Model file for the job. Use its own axes, mm. A direction names the side the tool comes from. Give positions to 0.01 mm unless a question says otherwise; leave off trailing zeros. Loops run counter-clockwise (first coordinate to the right, second up) from the corner with the lowest first, then second, coordinate; pieces in that order, holes last. Notation, with made-up numbers: (-34.5, 72.5) - (16.5, 72.5) arc R31 ccw to (16.5, 109.5) - close; hole circle Ø1 at (9, -8). An arc over 180 degrees is marked (long way). Answer as CSV lines item,"result". Start each with the question number.
Item 1: Pull direction X, two halves, no side cores. Call faces 4 (the flat face through (0.25, 8, 1.6)), 5 (the cylindrical face through (-2.723, -0.637, 5.507)), 6 (the cylindrical face through (8, -1.72, 4.15)), 7 (the flat face through (1, 1, 6)): pulls with the +X half, pulls with the -X half, needs draft (parallel to the pull), parting line crosses it, or undercut.
Item 2: Drill centre lines: L1, parallel to Z at x = -0.75, y = -3; L2, parallel to X at y = -1.75, z = 3.1; L3, parallel to Y at x = 2, z = 4.4. Where is each one in solid material? Low to high. Write a range as from..to.
Item 3: Pin check, flat tips, straight feed: pin 1 (3 mm diameter, centred on y = 6, z = 2.5, fed in from +X); pin 2 (1 mm diameter, centred on x = 1, z = 2.5, fed in from -Y); pin 3 (5 mm diameter, centred on x = -1, y = -2, fed in from +Z); pin 4 (1 mm diameter, centred on y = 2, z = 3, fed in from +X). Stop position of each tip, or through.
Item 4: Saw through at A-A on y = 6.75. Give the cut face in (x, z), plus the area to 3 significant figures.
Item 5: Saw through at D-D on z = 0.5. Give the cut face in (x, y).
Item 6: Saw through at C-C on z = 3. Give the cut face in (x, y), plus the area to 3 significant figures.
Item 7: Tool access for faces 1 (the flat face through (2.3, -1, 3)), 2 (the flat face through (3.75, 2, 3)), 3 (the flat face through (-3.75, 3, 3)): list every direction of +Z, -Z, +X, -X, +Y, -Y with a clear straight run to the whole face (end or side of a thin tool).
from build123d import *

# Parameters (mm, degrees)
SKETCH_W        = 7.5
SKETCH_H        = 7.5
PAD_DEPTH       = 6
SKETCH001_W     = 4
SKETCH001_H     = 6
PAD001_DEPTH    = 6
SKETCH002_W     = 4
SKETCH002_H     = 6
PAD002_DEPTH    = 6
SKETCH003_R     = 1.7
HOLE_DEPTH      = 4
HOLE_TIPS_R     = 1.7
SKETCH004_R     = 1.7
HOLE001_DEPTH   = 4
HOLE001_TIPS_R  = 1.7
SKETCH005_W     = 6.05
SKETCH005_H     = 3.05
POCKET_DEPTH    = 6.05
SKETCH006_R     = 2
POCKET001_DEPTH = 1


with BuildPart() as part:
    # Sketch → Pad (new body)
    with BuildSketch(Plane.XY):
        Rectangle(SKETCH_W, SKETCH_H)
    extrude(amount=PAD_DEPTH)

    # Sketch001 (on Face2 of Pad) → Pad001 (join)
    with BuildSketch(Plane(origin=(0, 3.75, 0), x_dir=(-1, 0, 0), z_dir=(0, 1, 0))):
        with Locations((1.75, 3)):
            Rectangle(SKETCH001_W, SKETCH001_H)
    extrude(amount=PAD001_DEPTH)

    # Sketch002 (on Face2 of Pad001) → Pad002 (join)
    with BuildSketch(Plane.YZ.offset(3.75)):
        with Locations((-1.75, 3)):
            Rectangle(SKETCH002_W, SKETCH002_H)
    extrude(amount=PAD002_DEPTH)

    # Sketch003 (on Face6 of Pad002) → Hole (cut)
    with BuildSketch(Plane(origin=(0, 0.25, 0), x_dir=(-1, 0, 0), z_dir=(0, 1, 0))):
        with Locations((-6.75, 3)):
            Circle(SKETCH003_R)
    extrude(amount=-HOLE_DEPTH, mode=Mode.SUBTRACT)

    # Hole tips → Hole tip 1 section 0
    with BuildSketch(Plane(origin=(0, -3.75, 0), x_dir=(-1, 0, 0), z_dir=(0, 1, 0)), mode=Mode.PRIVATE) as hole_tip_1_s0:
        with Locations((-6.75, 3)):
            Circle(HOLE_TIPS_R)
    loft([hole_tip_1_s0.sketch, Vertex(6.75, -4.771463, 3)], mode=Mode.SUBTRACT)

    # Sketch004 (on Face11 of Hole) → Hole001 (cut)
    with BuildSketch(Plane.YZ.offset(0.25)):
        with Locations((6.75, 3)):
            Circle(SKETCH004_R)
    extrude(amount=-HOLE001_DEPTH, mode=Mode.SUBTRACT)

    # Hole001 tips → Hole001 tip 1 section 0
    with BuildSketch(Plane.YZ.offset(-3.75), mode=Mode.PRIVATE) as hole001_tip_1_s0:
        with Locations((6.75, 3)):
            Circle(HOLE001_TIPS_R)
    loft([hole001_tip_1_s0.sketch, Vertex(-4.771463, 6.75, 3)], mode=Mode.SUBTRACT)

    # Sketch005 (on Face2 of Hole001) → Pocket (cut)
    with BuildSketch(Plane.XZ.offset(3.75)):
        with Locations((-0.725, 3.475)):
            Rectangle(SKETCH005_W, SKETCH005_H)
    extrude(amount=-POCKET_DEPTH, mode=Mode.SUBTRACT)

    # Sketch006 (on Face4 of Pocket) → Pocket001 (cut)
    with BuildSketch(Plane.XY.offset(6)):
        with Locations((-0.725, -0.725)):
            Circle(SKETCH006_R)
    extrude(amount=-POCKET001_DEPTH, mode=Mode.SUBTRACT)


solid = part.part
Responses:
1,face 4,"pulls with the +X half"
1,face 5,"undercut"
1,face 6,"undercut"
1,face 7,"needs draft"
2,L1,"0..1.95, 5..6"
2,L2,"2.3..5.05, 8.45..9.75"
2,L3,"2.3..3.75"
3,pin 1,"x = 0.25"
3,pin 2,"y = 2.3"
3,pin 3,"z = 6"
3,pin 4,"x = 3.75"
4,outline,"(-3.75, 0) - (0.25, 0) - (0.25, 1.3) - (-3.75, 1.3) - close; (-3.75, 4.7) - (0.25, 4.7) - (0.25, 6) - (-3.75, 6) - close"
4,area,"10.4 mm2"
5,outline,"(-3.75, -3.75) - (9.75, -3.75) - (9.75, 0.25) - (3.75, 0.25) - (3.75, 3.75) - (0.25, 3.75) - (0.25, 9.75) - (-3.75, 9.75) - close"
6,outline,"(-3.75, 2.3) - (2.3, 2.3) - (2.3, -3.75) - (5.05, -3.75) - (5.05, 0.25) - (3.75, 0.25) - (3.75, 3.75) - (0.25, 3.75) - (0.25, 5.05) - (-3.75, 5.05) - close; (-3.75, 8.45) - (0.25, 8.45) - (0.25, 9.75) - (-3.75, 9.75) - close; (8.45, -3.75) - (9.75, -3.75) - (9.75, 0.25) - (8.45, 0.25) - close"
6,area,"40.4 mm2"
7,face 1,"-X, -Y"
7,face 2,"+Z, -Z, +X, +Y"
7,face 3,"+Z, -Z, -X, +Y, -Y"
